```python
from build123d import *

# Parameters (mm, degrees)
SKETCH1_R           = 20
SKETCH1_R_2         = 4
SKETCH1_R_3         = 1.75
SKETCH1_R_4         = 1.5
BOSS_EXTRUDE1_DEPTH = 6
MOVE_FACE2_BY       = 0.08
MOVE_FACE2_2_BY     = 0.08
MOVE_FACE2_3_BY     = 0.08
MOVE_FACE2_4_BY     = 0.08
MOVE_FACE2_5_BY     = 0.08
MOVE_FACE2_6_BY     = 0.08
MOVE_FACE2_7_BY     = 0.08
MOVE_FACE2_8_BY     = 0.08
MOVE_FACE2_9_BY     = 0.08


with BuildPart() as part:
    # Sketch1 → Boss-Extrude1 (new body)
    with BuildSketch(Plane.XY):
        Circle(SKETCH1_R)
        Circle(SKETCH1_R_2, mode=Mode.SUBTRACT)
        with Locations((0, 15)):
            Circle(SKETCH1_R_3, mode=Mode.SUBTRACT)
        with Locations((10.606601718, 10.606601718)):
            Circle(SKETCH1_R_4, mode=Mode.SUBTRACT)
        with Locations((15, 0)):
            Circle(SKETCH1_R_3, mode=Mode.SUBTRACT)
        with Locations((10.606601718, -10.606601718)):
            Circle(SKETCH1_R_4, mode=Mode.SUBTRACT)
        with Locations((0, -15)):
            Circle(SKETCH1_R_3, mode=Mode.SUBTRACT)
        with Locations((-10.606601718, -10.606601718)):
            Circle(SKETCH1_R_4, mode=Mode.SUBTRACT)
        with Locations((-15, 0)):
            Circle(SKETCH1_R_3, mode=Mode.SUBTRACT)
        with Locations((-10.606601718, 10.606601718)):
            Circle(SKETCH1_R_4, mode=Mode.SUBTRACT)
    extrude(amount=BOSS_EXTRUDE1_DEPTH)

    # Move Face2: a curved face moved outward by 0.08
    add(Solid.thicken(part.faces().sort_by_distance((-4, 0, 3))[0], MOVE_FACE2_BY))

    # Move Face2 2: a curved face moved outward by 0.08
    add(Solid.thicken(part.faces().sort_by_distance((-1.75, 15, 3))[0], MOVE_FACE2_2_BY))

    # Move Face2 3: a curved face moved outward by 0.08
    add(Solid.thicken(part.faces().sort_by_distance((9.106601718, 10.606601718, 3))[0], MOVE_FACE2_3_BY))

    # Move Face2 4: a curved face moved outward by 0.08
    add(Solid.thicken(part.faces().sort_by_distance((13.25, 0, 3))[0], MOVE_FACE2_4_BY))

    # Move Face2 5: a curved face moved outward by 0.08
    add(Solid.thicken(part.faces().sort_by_distance((9.106601718, -10.606601718, 3))[0], MOVE_FACE2_5_BY))

    # Move Face2 6: a curved face moved outward by 0.08
    add(Solid.thicken(part.faces().sort_by_distance((-1.75, -15, 3))[0], MOVE_FACE2_6_BY))

    # Move Face2 7: a curved face moved outward by 0.08
    add(Solid.thicken(part.faces().sort_by_distance((-12.106601718, -10.606601718, 3))[0], MOVE_FACE2_7_BY))

    # Move Face2 8: a curved face moved outward by 0.08
    add(Solid.thicken(part.faces().sort_by_distance((-16.75, 0, 3))[0], MOVE_FACE2_8_BY))

    # Move Face2 9: a curved face moved outward by 0.08
    add(Solid.thicken(part.faces().sort_by_distance((-12.106601718, 10.606601718, 3))[0], MOVE_FACE2_9_BY))


solid = part.part
```
Model file for the job. Use its own axes, mm. Coordinates: 2 decimals unless noted, no trailing zeros. Order: outer loops, then holes, each group sorted by start corner. A loop starts at its lowest first (then second) coordinate and runs counter-clockwise, first axis right, second up. Notation, with made-up numbers: (47.5, 8.25) - (58.5, 8.25) arc R26 ccw to (58.5, 22.25) - close; hole circle Ø7 at (-20.5, -14). An arc over 180 degrees is marked (long way). Return JSON: item names as keys, results as strings. Group by question number.
1) Saw through at A-A, the plane x = 0. Write the cut outline in (y, z).
2) Saw through at C-C, the plane x = 14.5. Write the cut outline in (y, z).
3) Probe line 1 (Y direction, x = 0, z = 4.1); line 2 (X direction, y = 10, z = 2.3); line 3 (Y direction, x = -10.5, z = 0.45). List the from-to ranges inside material, lowest first. Write a range as from..to.
4) Saw through at D-D, the plane z = 3.45. Count the separate pieces of the cut face and the enclosed holes in it, plus the area to 3 significant figures.
5) Mould opens along Y. For faces 1 (the cylindrical face through (-0.85, -3.827, 2.958)), 2 (the flat face through (4.2, 0.3, 6)), 3 (the cylindrical face through (-16.325, -1.016, 2.958)), 4 (the cylindrical face through (-4.336, -19.524, 2.958)) say: released by +Y, released by -Y, zero draft, split by the parting line, or undercut.
6) Flat gauge pins, fed straight in: P1, Ø1, axis at x = -10.5, z = 5, coming from the -Y side; P2, Ø1.5, axis at x = -11, z = 4.5, coming from the +Y side; P3, Ø3, axis at x = -13.5, z = 4.5, coming from the -Y side. Where does each tip first touch, or does it go through?
Values found:
{
 "1": {"outline": "(-20, 0) - (-16.67, 0) - (-16.67, 6) - (-20, 6) - close; (-13.33, 0) - (-3.92, 0) - (-3.92, 6) - (-13.33, 6) - close; (3.92, 0) - (13.33, 0) - (13.33, 6) - (3.92, 6) - close; (16.67, 0) - (20, 0) - (20, 6) - (16.67, 6) - close"},
 "2": {"outline": "(-13.77, 0) - (-1.59, 0) - (-1.59, 6) - (-13.77, 6) - close; (1.59, 0) - (13.77, 0) - (13.77, 6) - (1.59, 6) - close"},
 "3": {"line 1": "y = -20..-16.67, -13.33..-3.92, 3.92..13.33, 16.67..20", "line 2": "x = -17.32..-11.89, -9.32..9.32, 11.89..17.32", "line 3": "y = -17.02..-12.02, -9.19..9.19, 12.02..17.02"},
 "4": {"separate pieces": "1", "enclosed holes": "9", "area": "1,150 mm²"},
 "5": {"face 1": "undercut", "face 2": "zero draft", "face 3": "undercut", "face 4": "split by the parting line"},
 "6": {"P1": "stops at y = -17.32", "P2": "stops at y = 17.17", "P3": "stops at y = -16"}
}
